Job drawing, mm, ordinate dimensions from the low corner. One solid piece. A direction names the side the tool comes from. Round coordinates to 2 decimals unless told otherwise and drop trailing zeros. Write each loop counter-clockwise with the first axis right and the second up, starting at its lowest first coordinate (ties: lowest second). Pieces come first, ordered by that corner, then holes. Notation, with made-up numbers: M 68,2 L 92,2 A25 cw 92,18 Z; hole C 79,55.25 d6. An arc over 180 degrees is marked long. One line per item, written item: value. Start each with the question number.
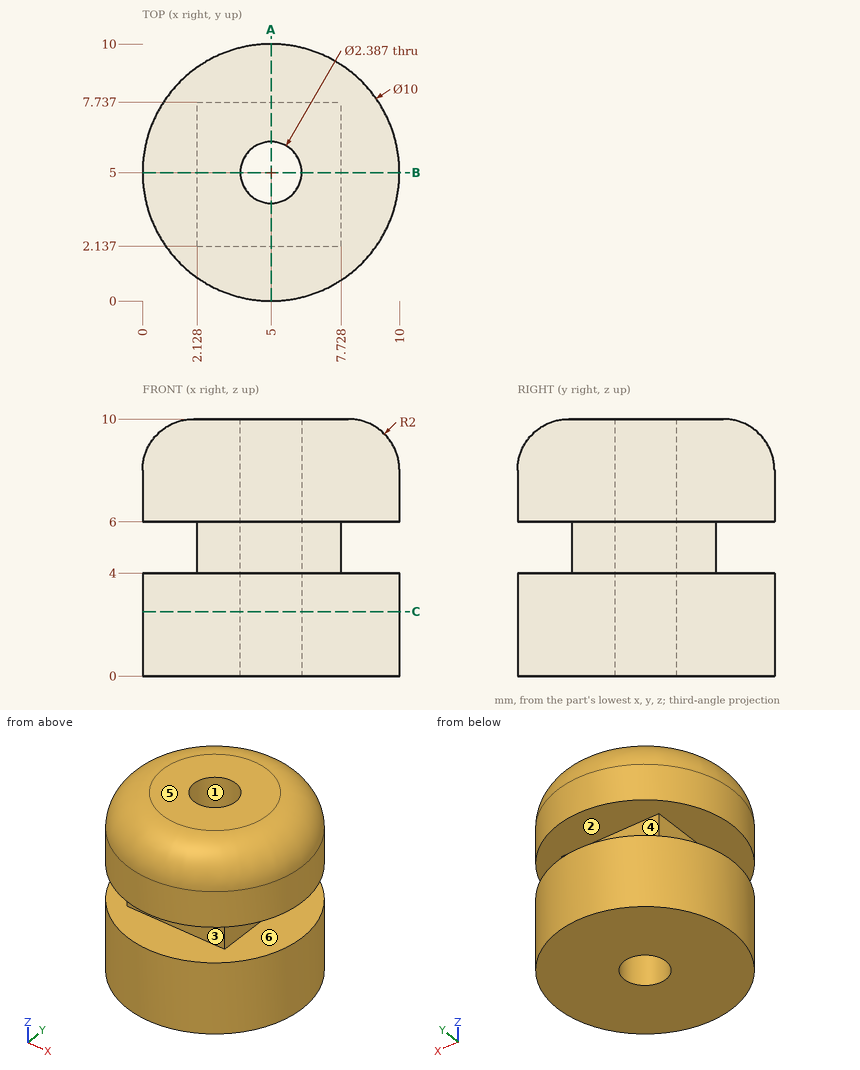
Item 1: Two-plate mould, pull along Y, no slides. Class the marked faces 1, 2, 3 and 4: pulls with the +Y half, pulls with the -Y half, needs draft (parallel to the pull), parting line crosses it, or undercut.
Item 2: Cut at A-A, the plane x = 5. Write the cut outline in (y, z).
Item 3: Which spindle directions (+Z, -Z, +X, -X, +Y, -Y) get a long thin tool onto all of the face, cutting with end or side? Do the marked faces 5 and 6. Say none if no direction does.
Item 4: Drill centre lines: line 1 (Y direction, x = 5, z = 3); line 2 (Z direction, x = 4, y = 1.75); line 3 (Y direction, x = 5.75, z = 2.75). Where is each one in solid material? Low to high.
Item 5: Cut at C-C, the plane z = 2.5. Write the cut outline in (x, y).
Item 6: Drop flat-ended pins along their axis: pin 1 (0.6 mm diameter, centred on x = 4, z = 5.5, fed in from -Y); pin 2 (0.6 mm diameter, centred on y = 5, z = 4.5, fed in from +X); pin 3 (1.6 mm diameter, centred on y = 4, z = 5.5, fed in from -X). Give the stop position or say it passes through.
Item 7: Cut at B-B, the plane y = 5. Write the cut outline in (x, z), plus the area to 3 significant figures.
Computed values:
1. face 1: undercut
1. face 2: needs draft
1. face 3: pulls with the -Y half
1. face 4: pulls with the +Y half
2. outline: M 0,0 L 3.81,0 L 3.81,10 L 2,10 A2 ccw 0,8 L 0,6 L 2.14,6 L 2.14,4 L 0,4 Z; M 6.19,0 L 10,0 L 10,4 L 7.74,4 L 7.74,6 L 10,6 L 10,8 A2 ccw 8,10 L 6.19,10 Z
3. face 5: +Z, +X, -X, +Y, -Y
3. face 6: none
4. line 1: y = 0 to 3.81, 6.19 to 10
4. line 2: z = 0 to 4, 6 to 9.96
4. line 3: y = 0.06 to 4.07, 5.93 to 9.94
5. outline: C 5,5 d10; hole C 5,5 d2.39
6. pin 1: stops at y = 2.14
6. pin 2: stops at x = 7.73
6. pin 3: stops at x = 0.01
7. outline: M 0,0 L 3.81,0 L 3.81,10 L 2,10 A2 ccw 0,8 L 0,6 L 2.13,6 L 2.13,4 L 0,4 Z; M 6.19,0 L 10,0 L 10,4 L 7.73,4 L 7.73,6 L 10,6 L 10,8 A2 ccw 8,10 L 6.19,10 Z
7. area: 65.6 mm2
